from build123d import *

# Parameters (mm, degrees)
BOSS_EXTRUDE1_DEPTH     = 4.5
CHAMFER2_SIZE           = 1
CHAMFER3_SIZE           = 1
CUT_EXTRUDE1_DEPTH      = 38.7458607
CUT_EXTRUDE1_DEPTH_BACK = 38.7458607
SKETCH2_R               = 2
SKETCH3_R               = 3
CUT_EXTRUDE4_DEPTH      = 13


with BuildPart() as part:
    # Sketch1 → Boss-Extrude1 (new, symmetric)
    with BuildSketch(Plane(origin=(0, 0, 0), x_dir=(1, 0, 0), z_dir=(0, 1, 0))):
        with BuildLine():
            Line((-0.75, 21), (0.75, 21))
            Line((0.75, 21), (0.75, 17.483921185))
            ThreePointArc((0.75, 17.483921185), (17.5, 0), (0.75, -17.483921185))
            Line((0.75, -17.483921185), (0.75, -26.489384666))
            ThreePointArc((0.75, -26.489384666), (0, 26.5), (-0.75, -26.489384666))
            Line((-0.75, -26.489384666), (-0.75, -17.483921185))
            ThreePointArc((-0.75, -17.483921185), (-17.5, 0), (-0.75, 17.483921185))
            Line((-0.75, 17.483921185), (-0.75, 21))
        make_face()
    extrude(amount=BOSS_EXTRUDE1_DEPTH, both=True)

    # Chamfer2
    chamfer2_edges = [part.edges().sort_by_distance(p)[0] for p in [
        (0, 4.5, -26.5),
        (-17.5, 4.5, 0),
        (17.5, 4.5, 0),
    ]]
    chamfer(chamfer2_edges, length=CHAMFER2_SIZE)

    # Chamfer3
    chamfer3_edges = [part.edges().sort_by_distance(p)[0] for p in [
        (0, -4.5, -26.5),
        (17.5, -4.5, 0),
        (-17.5, -4.5, 0),
    ]]
    chamfer(chamfer3_edges, length=CHAMFER3_SIZE)

    # Sketch2 → Cut-Extrude1 (cut, two sides: drawn at the far end of the back side and taken through both)
    with BuildSketch(Plane(origin=(0, 0, 0), x_dir=(0, 0, -1), z_dir=(1, 0, 0)).offset(-CUT_EXTRUDE1_DEPTH_BACK)):
        with Locations((-21.989789185, 0)):
            Circle(SKETCH2_R)
    extrude(amount=CUT_EXTRUDE1_DEPTH + CUT_EXTRUDE1_DEPTH_BACK, mode=Mode.SUBTRACT)

    # Sketch3 → Cut-Extrude4 (cut)
    with BuildSketch(Plane(origin=(20, 0, 0), x_dir=(0, 0, -1), z_dir=(1, 0, 0))):
        with Locations((-21.989789185, 0)):
            Circle(SKETCH3_R)
    cut_extrude4 = extrude(amount=-CUT_EXTRUDE4_DEPTH, mode=Mode.SUBTRACT)

    # Mirror3: Cut-Extrude4 across plane
    add(cut_extrude4.mirror(Plane(origin=(0, 0, 0), x_dir=(0, 0, 1), z_dir=(1, 0, 0))), mode=Mode.SUBTRACT)


solid = part.part
Part model, mm, in its own coordinate system. A direction names the side the tool comes from. Give positions to 0.01 mm unless a question says otherwise; leave off trailing zeros. Order: outer loops, then holes, each group sorted by start corner. A loop starts at its lowest first (then second) coordinate and runs counter-clockwise, first axis right, second up. Notation, with made-up numbers: (63, 34.5) -> (87, 34.5) arc R31 ccw to (87, 68.5) -> close; hole circle Ø2 at (-10.5, -21). An arc over 180 degrees is marked (long way). Use one line per item in the form item = value.
(1) Flat gauge pins, fed straight in: P1, Ø1.8, axis at y = 0, z = -20, coming from the -X side; P2, Ø1.8, axis at y = 0, z = -19.5, coming from the +X side; P3, Ø1.5, axis at y = -0.5, z = -21, coming from the -X side. Where does each tip first touch, or does it go through?
Solution:
P1 = -18.37
P2 = 18.88
P3 = -17.09
(2) Saw through at B-B (x = -4.5). Count the separate pieces of the cut face and the enclosed holes in it, then the cut area to 3 significant figures.
Solution:
separate_pieces = 2
enclosed_holes = 1
area = 149 mm²
(3) Pull direction X, two halves, no side cores. Call faces 1 (the face through (-13.3, -4.5, 13.1)), 2 (the face through (-7, -2, 21)), 3 (the face through (-18, 4, 0)), 4 (the face through (1.118, 4.34, -25.635)): +X half, -X half, draft (parallel to the pull), parting line (faces both ways), or undercut.
Solution:
face_1 = draft
face_2 = -X half
face_3 = undercut
face_4 = parting line
(4) Saw through at C-C (y = 0). Write the cut outline in (x, z), then the cut area to 3 significant figures.
Solution:
outline = (-18.48, 18.99) arc R26.5 ccw (long way) to (18.48, 18.99) -> (7, 18.99) -> (7, 19.99) -> (0.75, 19.99) -> (0.75, 17.48) arc R17.5 cw to (0.75, -17.48) -> (0.75, -21) -> (-0.75, -21) -> (-0.75, -17.48) arc R17.5 cw to (-0.75, 17.48) -> (-0.75, 19.99) -> (-7, 19.99) -> (-7, 18.99) -> close; (-8.82, 24.99) -> (-7, 24.99) -> (-7, 23.99) -> (-0.75, 23.99) -> (-0.75, 26.49) arc R26.5 ccw to start; (0.75, 23.99) -> (7, 23.99) -> (7, 24.99) -> (8.82, 24.99) arc R26.5 ccw to (0.75, 26.49) -> close
area = 1,090 mm²
(5) Tool access for faces 5 (the face through (11.55, 0.9, 19.13)), 6 (the face through (18, -4, 0)), 7 (the face through (0.75, 1, 24)), 8 (the face through (18, 4, 0)), 9 (the face through (-17.496, 0.049, 0.374)): list every direction of +Z, -Z, +X, -X, +Y, -Y with a clear straight run to the whole face (end or side of a thin tool).
Solution:
face_5 = +X
face_6 = -Y
face_7 = +Z, +Y, -Y
face_8 = +Y
face_9 = +Y, -Y
(6) Drill centre lines: line 1 (Y direction, x = -1, z = 22); line 2 (Z direction, x = 4.25, y = 0); line 3 (Z direction, x = -5, y = 0). Where is each one in solid material? Low to high. Write a range as from..to.
Solution:
line_1 = -4.5..-2, 2..4.5
line_2 = -26.16..-16.98, 16.98..19.99, 23.99..26.16
line_3 = -26.02..-16.77, 16.77..19.99, 23.99..26.02
(7) Saw through at A-A (z = 0). Write the cut outline in (x, y), then the cut area to 3 significant figures.
Solution:
outline = (-26.5, -3.5) -> (-25.5, -4.5) -> (-18.5, -4.5) -> (-17.5, -3.5) -> (-17.5, 3.5) -> (-18.5, 4.5) -> (-25.5, 4.5) -> (-26.5, 3.5) -> close; (17.5, -3.5) -> (18.5, -4.5) -> (25.5, -4.5) -> (26.5, -3.5) -> (26.5, 3.5) -> (25.5, 4.5) -> (18.5, 4.5) -> (17.5, 3.5) -> close
area = 158 mm²
